Check sheet for the modelled part. Datum: model origin and axes. Units: mm. Face numbers are marked on the shaded views. A direction names the side the tool comes from. Give positions to 0.01 mm unless a question says otherwise; leave off trailing zeros. Order: outer loops, then holes, each group sorted by start corner. A loop starts at its lowest first (then second) coordinate and runs counter-clockwise, first axis right, second up.
Item 1: Sectioned sample at C-C on y = 8.25. Record the boundary of the cut face in (x, z).
Item 2: Release check for a two-part mould opening along Z. For the marked faces 5, 6 and 7 record: released by +Z, released by -Z, zero draft, split by the parting line, or undercut.
Item 3: Gauge pin test, flat ends, axial feed: P1, Ø4, axis at x = 5.5, y = 5.5, coming from the +Z side; P2, Ø3, axis at x = 6.5, z = -12, coming from the +Y side; P3, Ø2, axis at x = 16.5, y = 8.5, coming from the -Z side. Record the tip position at first contact, or that the pin passes through.
Item 4: Sectioned sample at B-B on x = 8.89. Count the separate pieces of the cut face and the enclosed holes in it, and give its area (3 significant figures).
Item 5: Access from +Z, -Z, +X, -X, +Y, -Y to the whole of each face (thin tool, end or side, straight path). Record for the marked faces 1, 2, 3 and 4.
Item 6: Sectioned sample at A-A on y = 4. Record the boundary of the cut face in (x, z).
Item 7: Material ranges on line 1 along Z through (x, y) = (8.89, 1.45); line 2 along Z through (x, y) = (13.75, 5); line 3 along X through (y, z) = (1.5, -12), recorded low to high.
Item 8: Sectioned sample at D-D on x = 4.75. Record the boundary of the cut face in (y, z) (3 decimals).
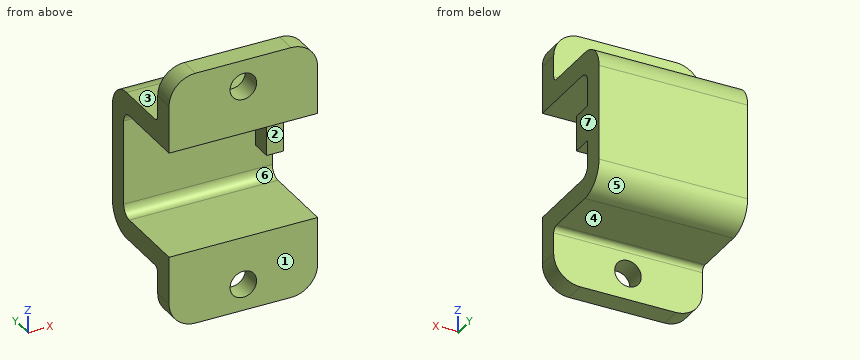
Autodesk Inventor part; units mm, degrees
ref_plane "YZ Plane" through (0, 0, 0) normal (1, 0, 0) x (0, 1, 0)
ref_plane "XZ Plane" through (0, 0, 0) normal (0, 1, 0) x (-1, 0, 0)
ref_plane "XY Plane" through (0, 0, 0) normal (0, 0, 1) x (1, 0, 0)
sketch "Sketch1" plane through (0, 0, 0) normal (1, 0, 0) x (0, 1, 0)
  line L0 (0, 15.24) -> (2.54, 15.24)
  line L1 (2.54, 15.24) -> (2.54, 8.89)
  line L2 (2.54, 8.89) -> (12.7, 8.89)
  line L3 (12.7, 8.89) -> (12.7, -8.89)
  line L4 (12.7, -8.89) -> (2.54, -8.89)
  line L5 (2.54, -8.89) -> (2.54, -15.24)
  line L6 (0, 15.24) -> (0, 6.35)
  line L7 (0, 6.35) -> (10.16, 6.35)
  line L8 (10.16, 6.35) -> (10.16, -6.35)
  line L9 (10.16, -6.35) -> (0, -6.35)
  line L10 (0, -6.35) -> (0, -15.24)
  line L11 (0, -15.24) -> (2.54, -15.24)
  point P0 (0, 0)
  dimension "d0" = 12.7
  dimension "d1" = 10.16
  dimension "d2" = 12.7
  dimension "d3" = 17.78
  dimension "d4" = 2.54
  dimension "d5" = 6.35
  dimension "d6" = 2.54
  dimension "d7" = 8.89
  dimension "d8" = 8.89
extrude "Extrusion1" add sketch "Sketch1" along normal blind 17.78
sketch "Sketch2" plane through (0, 10.16, -6.35) normal (0, -1, 0) x (1, 0, 0)
  line L0 (17.78, 8.4328) -> (15.748, 8.4328)
  line L1 (15.748, 8.4328) -> (15.748, 4.2164)
  line L2 (15.748, 4.2164) -> (17.78, 4.2164)
  line L3 (17.78, 4.2164) -> (17.78, 8.4328)
  line L4 (17.78, 12.7) -> (17.78, 0)
  line L5 (0, 0) -> (17.78, 0)
  point P0 (0, 6.35)
  dimension "d11" = 2.032
  dimension "d12" = 0
  dimension "d13" = 4.2164
  dimension "d14" = 4.2164
extrude "Extrusion2" add sketch "Sketch2" along normal blind 2.54
fillet "Fillet1" radius 1.27 2 edges at (8.89, 10.16, 6.35) (8.89, 10.16, -6.35)
fillet "Fillet2" radius 3.175 2 edges at (8.89, 12.7, 8.89) (8.89, 12.7, -8.89)
sketch "Sketch3" plane through (0, 2.54, 15.24) normal (0, 1, 0) x (1, 0, 0)
  circle A0 centre (8.89, 3.175) radius 1.5875
  circle A1 centre (8.89, 27.305) radius 1.5875
  line L0 (0, 24.13) -> (0, 30.48)
  line L1 (0, 0) -> (0, 6.35)
  line L2 (0, 0) -> (17.78, 0)
  line L3 (0, 30.48) -> (17.78, 30.48)
  point P0 (0, 15.24)
  dimension "d19" = 3.175
  dimension "d20" = 3.175
  dimension "d21" = 8.89
  dimension "d22" = 8.89
  dimension "d23" = 3.175
  dimension "d24" = 3.175
fillet "Fillet3" radius 3.175 4 edges at (17.78, 1.27, 15.24) (17.78, 1.27, -15.24) (0, 1.27, -15.24) (0, 1.27, 15.24)
extrude "Extrusion3" cut sketch "Sketch3" against normal blind 6.985
fillet "Fillet4" radius 0.635 2 edges at (8.89, 2.54, 8.89) (8.89, 2.54, -8.89)
properties part number "MotorCap"
Report:
1. outline: (0, -8.89) - (17.78, -8.89) - (17.78, -6.35) - (0, -6.35) - close; (0, 6.35) - (17.78, 6.35) - (17.78, 8.89) - (0, 8.89) - close; (15.75, -2.13) - (17.78, -2.13) - (17.78, 2.08) - (15.75, 2.08) - close
2. face 5: released by -Z
2. face 6: undercut
2. face 7: zero draft
3. P1: stops at z = 8.89
3. P2: stops at y = 2.54
3. P3: stops at z = -8.89
4. separate pieces: 3
4. enclosed holes: 0
4. area: 109 mm2
5. face 1: +Z, -Z, +X, -X, -Y
5. face 2: +X, -X, -Y
5. face 3: +Z, +X, -X, +Y
5. face 4: -Z, +X, -X, +Y
6. outline: (0, -8.89) - (17.78, -8.89) - (17.78, -6.35) - (0, -6.35) - close; (0, 6.35) - (17.78, 6.35) - (17.78, 8.89) - (0, 8.89) - close
7. line 1: z = -15.24 to -13.65, -10.48 to -6.35, 6.35 to 10.48, 13.65 to 15.24
7. line 2: z = -8.89 to -6.35, 6.35 to 8.89
7. line 3: x = 0 to 7.3, 10.48 to 17.78
8. outline: (0, -15.24) - (2.54, -15.24) - (2.54, -9.525) arc R0.635 cw to (3.175, -8.89) - (9.525, -8.89) arc R3.175 ccw to (12.7, -5.715) - (12.7, 5.715) arc R3.175 ccw to (9.525, 8.89) - (3.175, 8.89) arc R0.635 cw to (2.54, 9.525) - (2.54, 15.24) - (0, 15.24) - (0, 6.35) - (8.89, 6.35) arc R1.27 cw to (10.16, 5.08) - (10.16, -5.08) arc R1.27 cw to (8.89, -6.35) - (0, -6.35) - close
